The model under review builds one solid part; all positions refer to its coordinate system, in mm. Face numbers are marked on the shaded views. Coordinates: 2 decimals unless noted, no trailing zeros. Write each loop counter-clockwise with the first axis right and the second up, starting at its lowest first coordinate (ties: lowest second). Pieces come first, ordered by that corner, then holes.
1) Add section D-D, the plane x = -8.5. State the section outline as (y, z) points, then the cut area to 3 significant figures.
2) For line 1 (X direction, y = 0, z = 20); line 2 (Y direction, x = -1.5, z = 56), list the stretches that pass through material, from the lowest coordinate up.
3) Add section C-C, the plane x = -1.5. State the section outline as (y, z) points, then the cut area to 3 significant figures.
4) Add section B-B, the plane z = 16. State the section outline as (x, y) points, then the cut area to 3 significant figures.
5) For P1, Ø11, axis at x = 0, y = 0, coming from the -Z side; P2, Ø5, axis at y = 6, z = 16.5, coming from the -X side; P3, Ø1.5, axis at y = -3.5, z = 8, coming from the +X side; P4, Ø4, axis at x = 2.5, y = -7.5, coming from the +Z side, all flat-tipped, find the tip position at first contact; note any pin that passes through.
6) Mouldability with a two-part tool opening along Y and no side actions: class the marked faces 1, 2 and 3 as released by +Y, released by -Y, zero draft, split by the parting line, or undercut.
7) Add section A-A, the plane y = -1.5. State the section outline as (x, z) points.
Autodesk Inventor part; units mm, degrees
ref_plane "Start Plane" through (0, 0, -2.5789) normal (0, 0, 1) x (1, 0, 0)
ref_plane "End Plane" through (0, 0, 69.1479) normal (0, 0, 1) x (1, 0, 0)
ref_plane "Work Plane4" through (6.5224, -8.4419, 69.2424) normal (-0.0922, 0.1193, 0.9886) x (0.9957, 0.0055, 0.0922)
ref_plane "Start Plane" through (0, 0, -2.5789) normal (0, 0, 1) x (1, 0, 0)
ref_plane "End Plane" through (0, 0, 69.1479) normal (0, 0, 1) x (1, 0, 0)
sketch "Sketch" plane through (0, 0, 0) normal (0, 0, 1) x (1, 0, 0)
  circle A0 centre (0, 0) radius 6.9342
  circle A1 centre (0, 0) radius 10.668
  dimension "d0" = 21.336
  dimension "d1" = 3.7338
extrude "Body" add sketch "Sketch" along normal up to surface (71.7269 mm away) from surface at -2.5789
sketch "Sketch3" plane through (0, 0, 0) normal (0, 0, 1) x (1, 0, 0)
  line L0 (0, 0) -> (10, 0)
ref_plane "Work Plane3" through (0, 0, 0) normal (0, -1, 0) x (1, 0, 0)
sketch "Sketch4" plane through (0, 0, 0) normal (0, -1, 0) x (1, 0, 0)
  line L0 (-2, -2.5789) -> (12, -2.5789)
  line L1 (-2, 69.1479) -> (12, 69.1479)
  dimension "d7" = 71.7268
ref_plane "Work Plane4" through (6.5224, -8.4419, 69.2424) normal (-0.0922, 0.1193, 0.9886) x (0.9957, 0.0055, 0.0922)
split "Split1" plane through (6.5224, -8.4419, 69.2424) removes the side toward (-0.0922, 0.1193, 0.9886)
ref_plane "Work Plane5" through (-10.3791, -2.4658, -9.228) normal (0.6365, 0.1512, -0.7563) x (-0.6625, -0.395, -0.6365)
split "Split2" plane through (-10.3791, -2.4658, -9.228) removes the side toward (0.6365, 0.1512, -0.7563)
ref_plane "Work Plane6" through (0, -10.668, -2.5822) normal (0, 0.2353, -0.9719) x (1, 0, 0)
split "Split3" plane through (0, -10.668, -2.5822) removes the side toward (0, 0.2353, -0.9719)
ref_plane "Work Plane7" through (-9.0379, -5.6677, 73.9403) normal (0.432, 0.2709, 0.8602) x (0.8997, -0.0629, -0.432)
split "Split4" plane through (-9.0379, -5.6677, 73.9403) removes the side toward (0.432, 0.2709, 0.8602)
ref_plane "Work Plane8" through (8.1097, -16.9443, 26.4447) normal (0.1452, -0.9876, -0.059) x (0.0697, -0.0493, 0.9963)
sketch "Sketch5" plane through (8.1097, -16.9443, 26.4447) normal (0.1452, -0.9876, -0.059) x (0.0697, -0.0493, 0.9963)
  circle A0 centre (30.9821, 4.1171) radius 3
  point P0 (-27.7483, 3.8509)
hole "Hole1" at (6.2064, -19.0834, 57.5677) direction (-0.1452, 0.9876, 0.059) diameter 5.4 depth 20 tip angle 118
equation "\"d0\" = G_H"
equation "\"d1\" = G_T"
equation "\"d2\" = G_L"
equation "\"G_H\" = 21.336"
equation "\"G_T\" = 3.7338"
equation "\"G_L\" = 71.72685"
equation "\"G_OFFSET_START\" = 2.57893"
equation "\"G_OFFSET_END\" = 1.53222"
equation "\"d4\" = -G_OFFSET_START"
equation "\"d5\" = G_OFFSET_END + B_L"
equation "\"B_L\" = 67.61571"
properties part number "ANSI - 1/2 x 0.147 - 2.824" material "Steel, Mild"
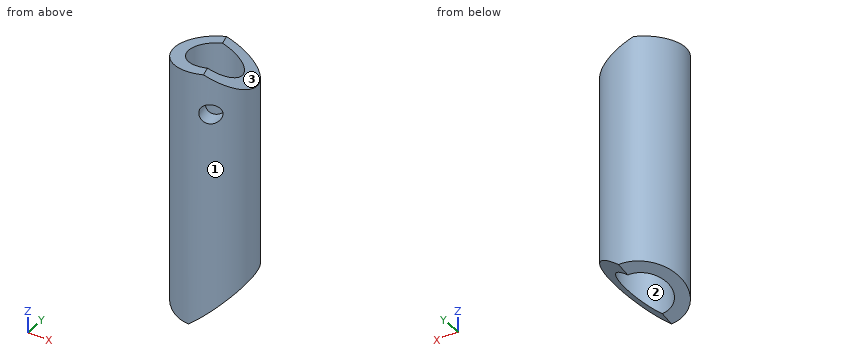
Geometry results:
1. outline: (-6.45, -1.56) - (6.45, 1.56) - (6.45, 66.04) - (-6.45, 67.6) - close
1. area: 862 mm2
2. line 1: x = -10.67 to -6.93, 6.93 to 10.67
2. line 2: y = -10.56 to -6.77, 6.77 to 10.56
3. outline: (-10.56, -2.56) - (-6.77, -1.64) - (-6.77, 68.29) - (-10.56, 68.75) - close; (6.77, 1.64) - (10.56, 2.56) - (10.56, 65.04) - (6.77, 66.24) - close
3. area: 509 mm2
4. outline: circle Ø21.34 at (0, 0); hole circle Ø13.87 at (0, 0)
4. area: 206 mm2
5. P1: passes through
5. P2: stops at x = -10.08
5. P3: stops at x = 10.3
5. P4: stops at z = 69.04
6. face 1: split by the parting line
6. face 2: undercut
6. face 3: released by +Y
7. outline: (-10.56, -0.36) - (-6.77, -0.36) - (-6.77, 67.16) - (-10.56, 66.81) - close; (6.77, 5.4) - (10.56, 8.59) - (10.56, 62.78) - (6.77, 64.69) - close
